CAD build for the part. Positions are in the model's coordinates, mm. A direction names the side the tool comes from. Coordinates: 2 decimals unless noted, no trailing zeros. Loops run counter-clockwise (first coordinate to the right, second up) from the corner with the lowest first, then second, coordinate; pieces in that order, holes last.
1) Saw through at B-B, the plane y = 49.2. Write the cut outline in (x, z), and give its area (3 significant figures).
2) Wall check: line 1 along Y through (x, z) = (-2.25, 3.8); line 2 along Y through (x, z) = (-3, 46); line 3 along Z through (x, y) = (-2, 31). Give the ranges that are in metal, low to high.
3) Two-plate mould, pull along Y, no slides. Class faces 3 (the flat face through (-4, 20, 0)), 4 (the cylindrical face through (25, -5, 25)), 5 (the cylindrical face through (-5.07, 48.224, 3.583)): +Y half, -Y half, draft (parallel to the pull), parting line (faces both ways), or undercut.
4) Saw through at C-C, the plane z = 31. Write the cut outline in (x, y).
5) Saw through at D-D, the plane y = 8. Write the cut outline in (x, z), and give its area (3 significant figures).
6) Which spindle directions (+Z, -Z, +X, -X, +Y, -Y) get a long thin tool onto all of the face, cutting with end or side? Do faces 1 (the flat face through (0, 30, 25)), 2 (the flat face through (-10, 25, 25)). Say none if no direction does.
7) Saw through at A-A, the plane x = -1. Write the cut outline in (y, z).
8) Pin check, flat tips, straight feed: pin 1 Ø2.5 at (y, z) = (31.4, 46.2) entering from +X; pin 2 Ø2 at (x, z) = (-2, 41.5) entering from +Y; pin 3 Ø8 at (x, z) = (20.5, 27) entering from +Y. Stop position of each tip, or through.
```python
from build123d import *

# Parameters (mm, degrees)
BOSS_EXTRUDE1_DEPTH = 50
SKETCH2_R           = 1
CUT_EXTRUDE1_DEPTH  = 10


with BuildPart() as part:
    # Sketch1 → Boss-Extrude1 (new body)
    with BuildSketch(Plane.XY):
        with BuildLine():
            Line((0, 60), (0, 0))
            Line((0, 0), (20, 0))
            ThreePointArc((20, 0), (25, -5), (20, -10))
            Line((20, -10), (-10, -10))
            Line((-10, -10), (-10, 60))
            ThreePointArc((-10, 60), (-5, 65), (0, 60))
        make_face()
    extrude(amount=BOSS_EXTRUDE1_DEPTH)

    # Sketch2 → Cut-Extrude1 (cut)
    with BuildSketch(Plane.ZY.offset(10)):
        with Locations((3.8, 31.4)):
            Circle(SKETCH2_R)
        with Locations((3.8, 49.2)):
            Circle(SKETCH2_R)
        with Locations((46.2, 31.4)):
            Circle(SKETCH2_R)
        with Locations(Location((46.2, 49.2, 0), (0, 0, 180))):
            Circle(SKETCH2_R)
    extrude(amount=-CUT_EXTRUDE1_DEPTH, mode=Mode.SUBTRACT)


solid = part.part
```
Data:
1. outline: (-10, 0) - (0, 0) - (0, 2.8) - (-10, 2.8) - close; (-10, 4.8) - (0, 4.8) - (0, 45.2) - (-10, 45.2) - close; (-10, 47.2) - (0, 47.2) - (0, 50) - (-10, 50) - close
1. area: 460 mm2
2. line 1: y = -10 to 30.4, 32.4 to 48.2, 50.2 to 64.18
2. line 2: y = -10 to 30.42, 32.38 to 48.22, 50.18 to 64.58
2. line 3: z = 0 to 2.88, 4.72 to 45.28, 47.12 to 50
3. face 3: draft
3. face 4: parting line
3. face 5: undercut
4. outline: (-10, -10) - (20, -10) arc R5 ccw to (20, 0) - (0, 0) - (0, 60) arc R5 ccw to (-10, 60) - close
5. outline: (-10, 0) - (0, 0) - (0, 50) - (-10, 50) - close
5. area: 500 mm2
6. face 1: +Z, -Z, +X, +Y
6. face 2: +Z, -Z, -X, +Y, -Y
7. outline: (-10, 0) - (63, 0) - (63, 50) - (-10, 50) - close; hole circle Ø2 at (31.4, 3.8); hole circle Ø2 at (31.4, 46.2); hole circle Ø2 at (49.2, 3.8); hole circle Ø2 at (49.2, 46.2)
8. pin 1: stops at x = 0
8. pin 2: stops at y = 64.58
8. pin 3: stops at y = 0
